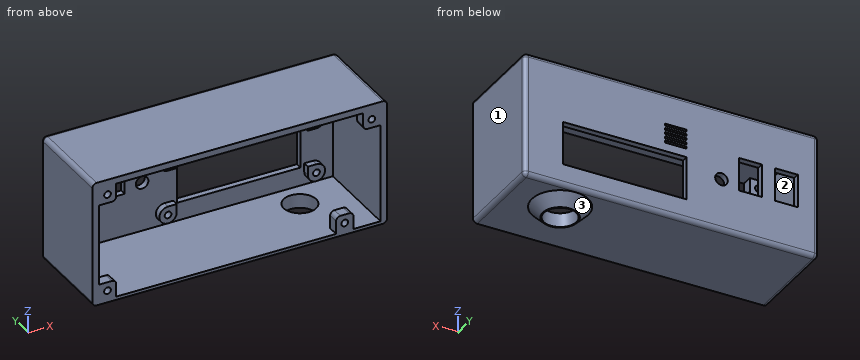
```python
from build123d import *

# Parameters (mm, degrees)
SKETCH1_W           = 172.72
SKETCH1_H           = 73.66
SKETCH1_R           = 3.683
SKETCH1_W_2         = 72.39
SKETCH1_H_2         = 25.4
SKETCH1_W_3         = 13.462
SKETCH1_H_3         = 19.558
BOSS_EXTRUDE1_DEPTH = 3.81
BOSS_EXTRUDE2_DEPTH = 3.81
SKETCH3_R           = 1.9685
CUT_EXTRUDE1_DEPTH  = 6.35
SKETCH4_W           = 172.72
SKETCH4_H           = 73.66
SKETCH4_W_2         = 165.1
SKETCH4_H_2         = 67.945
BOSS_EXTRUDE4_DEPTH = 50.8
FILLET1_R           = 2.54
SKETCH5_W           = 10.16
SKETCH5_H           = 10.16
BOSS_EXTRUDE5_DEPTH = 6.35
FILLET2_R           = 2.54
SKETCH6_R           = 1.9685
CUT_EXTRUDE2_DEPTH  = 6.35
SKETCH7_W           = 12.7
SKETCH7_H           = 1.27
CUT_EXTRUDE3_DEPTH  = 3.81
SKETCH8_R           = 9.525
CUT_EXTRUDE4_DEPTH  = 2.54
BOSS_EXTRUDE6_START = 6.35
SKETCH9_R           = 16.51
SKETCH9_R_2         = 9.525
BOSS_EXTRUDE6_DEPTH = 6.35
CHAMFER1_SIZE       = 6.35


with BuildPart() as part:
    # Sketch1 → Boss-Extrude1 (new body)
    with BuildSketch(Plane(origin=(0, 0, 0), x_dir=(1, 0, 0), z_dir=(0, 1, 0))):
        with Locations((86.36, 36.83)):
            Rectangle(SKETCH1_W, SKETCH1_H)
        with Locations(Location((57.023, 42.799, 0), (0, 0, 90))):
            Circle(SKETCH1_R, mode=Mode.SUBTRACT)
        with Locations((113.665, 48.26)):
            Rectangle(SKETCH1_W_2, SKETCH1_H_2, mode=Mode.SUBTRACT)
        with Locations((19.05, 36.83)):
            Rectangle(SKETCH1_W_3, SKETCH1_H_3, mode=Mode.SUBTRACT)
        with Locations((40.132, 36.83)):
            Rectangle(SKETCH1_W_3, SKETCH1_H_3, mode=Mode.SUBTRACT)
    extrude(amount=BOSS_EXTRUDE1_DEPTH)

    # Sketch2 → Boss-Extrude2 (add)
    with BuildSketch(Plane.XZ):
        with BuildLine():
            Line((70.1675, -37.465), (75.2475, -37.465))
            Line((75.2475, -37.465), (75.2475, -32.385))
            ThreePointArc((75.2475, -32.385), (66.575397552, -28.792897552), (70.1675, -37.465))
        make_face()
        with BuildLine():
            Line((70.1675, -59.055), (75.2475, -59.055))
            Line((75.2475, -59.055), (75.2475, -64.135))
            ThreePointArc((75.2475, -64.135), (66.575397552, -67.727102448), (70.1675, -59.055))
        make_face()
        with BuildLine():
            Line((152.0825, -32.385), (152.0825, -37.465))
            Line((152.0825, -37.465), (157.1625, -37.465))
            ThreePointArc((157.1625, -37.465), (160.754602448, -28.792897552), (152.0825, -32.385))
        make_face()
        with BuildLine():
            Line((152.0825, -64.135), (152.0825, -59.055))
            Line((152.0825, -59.055), (157.1625, -59.055))
            ThreePointArc((157.1625, -59.055), (160.754602448, -67.727102448), (152.0825, -64.135))
        make_face()
    extrude(amount=BOSS_EXTRUDE2_DEPTH)

    # Sketch3 → Cut-Extrude1 (cut)
    with BuildSketch(Plane.XZ.offset(3.81)):
        with Locations(Location((70.1675, -32.385, 0), (0, 0, 270))):
            Circle(SKETCH3_R)
        with Locations(Location((70.1675, -64.135, 0), (0, 0, 270))):
            Circle(SKETCH3_R)
        with Locations(Location((157.1625, -64.135, 0), (0, 0, 270))):
            Circle(SKETCH3_R)
        with Locations(Location((157.1625, -32.385, 0), (0, 0, 270))):
            Circle(SKETCH3_R)
    extrude(amount=-CUT_EXTRUDE1_DEPTH, mode=Mode.SUBTRACT)

    # Sketch4 → Boss-Extrude4 (add)
    with BuildSketch(Plane.XZ):
        with Locations((86.36, -36.83)):
            Rectangle(SKETCH4_W, SKETCH4_H)
        with Locations((86.36, -37.7825)):
            Rectangle(SKETCH4_W_2, SKETCH4_H_2, mode=Mode.SUBTRACT)
    extrude(amount=BOSS_EXTRUDE4_DEPTH)

    # Fillet1
    fillet1_edges = [part.edges().sort_by_distance(p)[0] for p in [
        (172.72, 3.81, -36.83),
        (86.36, 3.81, -73.66),
        (0, 3.81, -36.83),
        (0, -23.495, -73.66),
        (172.72, -23.495, -73.66),
        (172.72, -23.495, 0),
        (0, -23.495, 0),
        (86.36, 3.81, 0),
    ]]
    fillet(fillet1_edges, radius=FILLET1_R)

    # Sketch5 → Boss-Extrude5 (add)
    with BuildSketch(Plane.XZ.offset(50.8)):
        with Locations((8.89, -8.89)):
            Rectangle(SKETCH5_W, SKETCH5_H)
        with Locations((8.89, -66.675)):
            Rectangle(SKETCH5_W, SKETCH5_H)
        with Locations((163.83, -8.89)):
            Rectangle(SKETCH5_W, SKETCH5_H)
        with Locations((147.955, -66.675)):
            Rectangle(SKETCH5_W, SKETCH5_H)
    extrude(amount=-BOSS_EXTRUDE5_DEPTH)

    # Fillet2
    fillet2_edges = [part.edges().sort_by_distance(p)[0] for p in [
        (13.97, -47.625, -13.97),
        (13.97, -47.625, -61.595),
        (153.035, -47.625, -61.595),
        (142.875, -47.625, -61.595),
        (158.75, -47.625, -13.97),
    ]]
    fillet(fillet2_edges, radius=FILLET2_R)

    # Sketch6 → Cut-Extrude2 (cut)
    with BuildSketch(Plane.XZ.offset(50.8)):
        with Locations(Location((8.89, -66.675, 0), (0, 0, 270))):
            Circle(SKETCH6_R)
        with Locations(Location((8.89, -8.89, 0), (0, 0, 270))):
            Circle(SKETCH6_R)
        with Locations(Location((163.83, -8.89, 0), (0, 0, 270))):
            Circle(SKETCH6_R)
        with Locations(Location((147.955, -66.675, 0), (0, 0, 270))):
            Circle(SKETCH6_R)
    extrude(amount=-CUT_EXTRUDE2_DEPTH, mode=Mode.SUBTRACT)

    # Sketch7 → Cut-Extrude3 (cut)
    with BuildSketch(Plane(origin=(0, 3.81, 0), x_dir=(1, 0, 0), z_dir=(0, 1, 0))):
        with Locations((83.82, 29.845)):
            Rectangle(SKETCH7_W, SKETCH7_H)
        with Locations((83.82, 27.305)):
            Rectangle(SKETCH7_W, SKETCH7_H)
        with Locations((83.82, 24.765)):
            Rectangle(SKETCH7_W, SKETCH7_H)
        with Locations((83.82, 22.225)):
            Rectangle(SKETCH7_W, SKETCH7_H)
        with Locations((83.82, 19.685)):
            Rectangle(SKETCH7_W, SKETCH7_H)
    extrude(amount=-CUT_EXTRUDE3_DEPTH, mode=Mode.SUBTRACT)

    # Sketch8 → Cut-Extrude4 (cut)
    with BuildSketch(Plane(origin=(0, 0, -73.66), x_dir=(-1, 0, 0), z_dir=(0, 0, -1))):
        with Locations((-140.97, -15.621)):
            Circle(SKETCH8_R)
    extrude(amount=-CUT_EXTRUDE4_DEPTH, mode=Mode.SUBTRACT)

    # Sketch9 → Boss-Extrude6 (add)
    with BuildSketch(Plane(origin=(0, 0, -73.66), x_dir=(-1, 0, 0), z_dir=(0, 0, -1)).offset(BOSS_EXTRUDE6_START)):
        with Locations(Location((-140.97, -15.621, 0), (0, 0, 180))):
            Circle(SKETCH9_R)
        with Locations((-140.97, -15.621)):
            Circle(SKETCH9_R_2, mode=Mode.SUBTRACT)
    extrude(amount=-BOSS_EXTRUDE6_DEPTH)

    # Chamfer1
    chamfer1_edges = [part.edges().sort_by_distance(p)[0] for p in [
        (124.46, -15.621, -80.01),
    ]]
    chamfer(chamfer1_edges, length=CHAMFER1_SIZE - 0.0001)  # a hair under: the kernel refuses the full size


solid = part.part
```
Input: part model. Units: mm. Frame: model coordinates. Face numbers are marked on the shaded views. Round coordinates to 2 decimals unless told otherwise and drop trailing zeros. Order: outer loops, then holes, each group sorted by start corner. A loop starts at its lowest first (then second) coordinate and runs counter-clockwise, first axis right, second up. Notation, with made-up numbers: (18, 0.5) - (37, 0.5) arc R35 ccw to (37, 38.5) - close; hole circle Ø8 at (16, 57). An arc over 180 degrees is marked (long way). One line per question, with ' | ' between items. Start each with the question number.
1) Cut plane D-D, the plane y = -34. Return the cut outline in (x, z) (3 decimals).
2) Cut plane A-A, the plane x = 106. Return the cut outline in (y, z) (3 decimals).
3) Cut plane C-C, the plane x = 8.89. Give the number of separate pieces and of enclosed holes in the cut face, then the cut area to 3 significant figures.
4) Pull-direction query (Z, two-part tool) for the marked faces 1, 2 and 3; classes: +Z half, -Z half, draft (parallel to the pull), parting line (faces both ways), or undercut.
5) Cut plane B-B, the plane z = -8.89. Return the cut outline in (x, y), then the cut area to 3 significant figures.
6) Ray query, probe 1 along Z at (x, y) = (163.83, -47.25) (1 decimal); probe 2 along X at (y, z) = (-46, -8.89); probe 3 along Z at (x, y) = (58, -44) (3 decimals). Return the intervals inside material, ascending.
7) Contact query for flat-ended pins moving along their axis: P1, Ø2.5, axis at x = 157.16, z = -64.14, coming from the -Y side; P2, Ø5, axis at x = 165, y = -47.5, coming from the -Z side; P3, Ø4, axis at x = 69, z = -57.5, coming from the -Y side; P4, Ø1, axis at y = 1.5, z = -19.5, coming from the -X side. Output: stop coordinate, or through.
Worked out:
1) outline: (0, -71.12) arc R2.54 ccw to (2.54, -73.66) - (170.18, -73.66) arc R2.54 ccw to (172.72, -71.12) - (172.72, -2.54) arc R2.54 ccw to (170.18, 0) - (2.54, 0) arc R2.54 ccw to (0, -2.54) - close; hole (3.81, -71.755) - (168.91, -71.755) - (168.91, -3.81) - (3.81, -3.81) - close
2) outline: (-50.8, -73.66) - (1.27, -73.66) arc R2.54 ccw to (3.81, -71.12) - (3.81, -60.96) - (0, -60.96) - (0, -71.755) - (-50.8, -71.755) - close; (-50.8, -3.81) - (0, -3.81) - (0, -35.56) - (3.81, -35.56) - (3.81, -2.54) arc R2.54 ccw to (1.27, 0) - (-50.8, 0) - close
3) separate pieces: 3 | enclosed holes: 0 | area: 647 mm^2
4) face 1: draft | face 2: undercut | face 3: -Z half
5) outline: (0, -50.8) - (6.92, -50.8) - (6.92, -44.45) - (3.81, -44.45) - (3.81, 0) - (168.91, 0) - (168.91, -44.45) - (165.8, -44.45) - (165.8, -50.8) - (172.72, -50.8) - (172.72, 1.27) arc R2.54 ccw to (170.18, 3.81) - (2.54, 3.81) arc R2.54 ccw to (0, 1.27) - close; (10.86, -50.8) - (13.97, -50.8) - (13.97, -44.45) - (10.86, -44.45) - close; (158.75, -50.8) - (161.86, -50.8) - (161.86, -44.45) - (158.75, -44.45) - close | area: 1,120 mm^2
6) probe 1: z = -73.7 to -71.8, -14 to -10.9, -6.9 to 0 | probe 2: x = 0 to 6.92, 10.86 to 13.97, 158.75 to 161.86, 165.8 to 172.72 | probe 3: z = -73.66 to -71.755, -3.81 to 0
7) P1: stops at y = 2.54 | P2: stops at z = -73.66 | P3: stops at y = -3.81 | P4: stops at x = 0
